Source: three-view drawing plus pictorial views. Frame: mm from the lowest corner of the part. A direction names the side the tool comes from. Give positions to 0.01 mm unless a question says otherwise; leave off trailing zeros. Order: outer loops, then holes, each group sorted by start corner. A loop starts at its lowest first (then second) coordinate and runs counter-clockwise, first axis right, second up. Notation, with made-up numbers: (60, 41) -> (101, 41) arc R23 ccw to (101, 77) -> close; hole circle Ø10 at (65.5, 33.5). An arc over 180 degrees is marked (long way). Use a Markdown table: item, result. Add a question column.
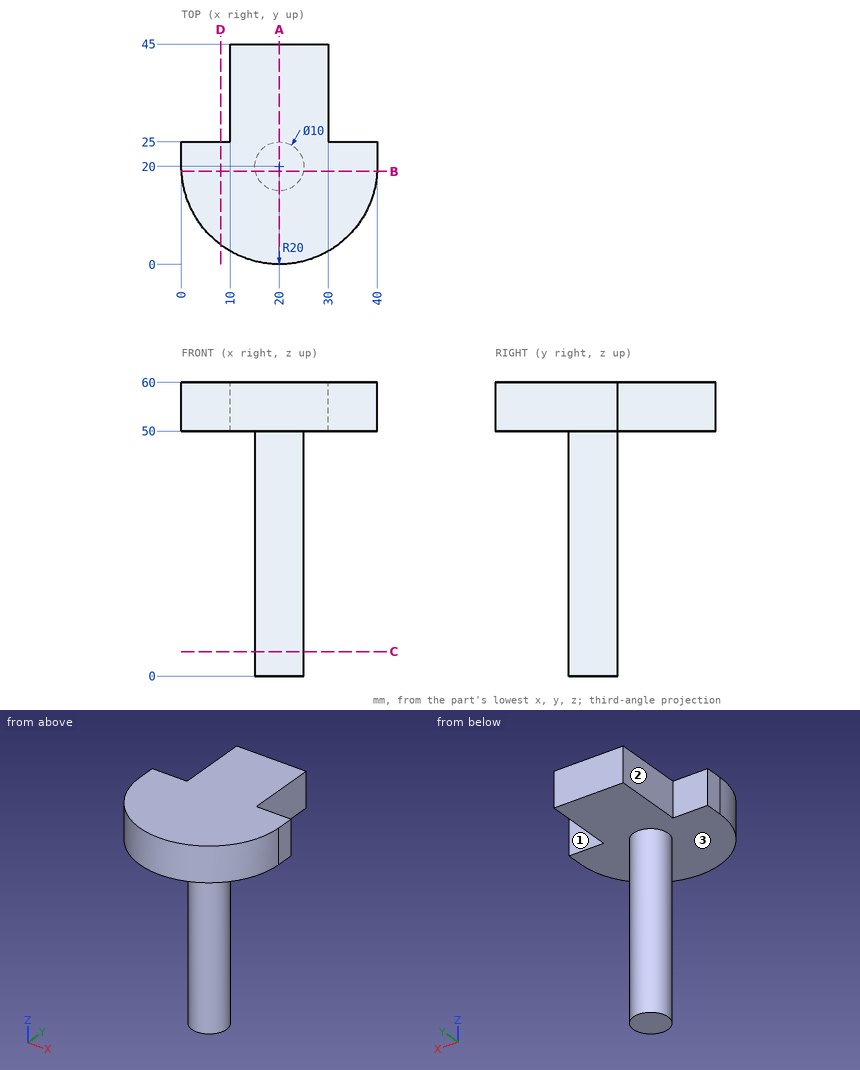
Q1. Access query for the marked faces 1, 2 and 3. Directions: +Z, -Z, +X, -X, +Y, -Y. A direction counts if a zero-diameter tool reaches every point of the face in a straight line with its end or side. Return the directions, or none.
Q2. Ray query, line 1 (Z direction, x = 38, y = 18.5); line 2 (X direction, y = 42.5, z = 57.5); line 3 (X direction, y = 17, z = 26). Return the intervals inside material, ascending.
Q3. Section query C-C (z = 5). Return loops of the section in (x, y).
Q4. Section query D-D (x = 8). Return loops of the section in (y, z), plus the area to 3 significant figures.
Q5. Section query B-B (y = 19). Return loops of the section in (x, z), plus the area to 3 significant figures.
Q6. Section query A-A (x = 20). Return loops of the section in (y, z), plus the area to 3 significant figures.
Q7. First-contact query: pin 1 (4 mm diameter, centred on x = 20.5, z = 7, fed in from +Y); pin 2 (11 mm diameter, centred on y = 38.5, z = 56, fed in from +X); pin 3 (5 mm diameter, centred on y = 31, z = 54.5, fed in from -X). Flat tips, straight axial feed; report the tip coordinate or a pass-through.
Solution:
| question | item | result |
|---|---|---|
| 1 | face 1 | +Z, -Z, +X, +Y |
| 1 | face 2 | +Z, -Z, -X, +Y |
| 1 | face 3 | -Z |
| 2 | line 1 | z = 50 to 60 |
| 2 | line 2 | x = 10 to 30 |
| 2 | line 3 | x = 16 to 24 |
| 3 | outline | circle Ø10 at (20, 20) |
| 4 | outline | (4, 50) -> (25, 50) -> (25, 60) -> (4, 60) -> close |
| 4 | area | 210 mm² |
| 5 | outline | (0.03, 50) -> (15.1, 50) -> (15.1, 0) -> (24.9, 0) -> (24.9, 50) -> (39.97, 50) -> (39.97, 60) -> (0.03, 60) -> close |
| 5 | area | 889 mm² |
| 6 | outline | (0, 50) -> (15, 50) -> (15, 0) -> (25, 0) -> (25, 50) -> (45, 50) -> (45, 60) -> (0, 60) -> close |
| 6 | area | 950 mm² |
| 7 | pin 1 | stops at y = 25 |
| 7 | pin 2 | stops at x = 30 |
| 7 | pin 3 | stops at x = 10 |
